Part model, mm, in its own coordinate system. Face numbers are marked on the shaded views. A direction names the side the tool comes from. Coordinates: 2 decimals unless noted, no trailing zeros. Write each loop counter-clockwise with the first axis right and the second up, starting at its lowest first coordinate (ties: lowest second). Pieces come first, ordered by that corner, then holes. Notation, with made-up numbers: M 19,0.5 L 51,0.5 A14 ccw 51,17.5 Z; hole C 79,8 d10. An arc over 180 degrees is marked long. Use a Markdown table: item, result. Add a question column.
Q1. Pin check, flat tip, straight feed: pin 1 Ø4 at (x, y) = (4.57, 10.04) entering from +Z. Stop position of the tip, or through.
Q2. Slice it at A-A on y = 2.96. Write the cut outline in (x, z).
Q3. Slice it at C-C on y = 22.61. Write the cut outline in (x, z).
Q4. Slice it at B-B on z = -1.7. Write the cut outline in (x, y).
Q5. Slice it at D-D on z = -0.35. Write the cut outline in (x, y), then the cut area to 3 significant figures.
Q6. Mould opens along Y. For the marked faces 3, 4, 5 and 6 say: released by +Y, released by -Y, zero draft, split by the parting line, or undercut.
Q7. Tool access for the marked faces 1 and 2: list every direction of +Z, -Z, +X, -X, +Y, -Y with a clear straight run to the whole face (end or side of a thin tool).
Q8. Wall check: L1, parallel to X at y = 11.75, z = -0.3; L2, parallel to X at y = 22.5, z = -1.75; L3, parallel to Y at x = 15, z = -1.65. Give the ranges that are in metal, low to high. Write a range as from..to.
from build123d import *

# Parameters (mm, degrees)
SKETCH1_W                                       = 20
SKETCH1_H                                       = 29.11
SKETCH1_R                                       = 1.5
SKETCH1_R_2                                     = 1.2
SKETCH1_R_3                                     = 5
BOSS_EXTRUDE2_DEPTH                             = 3.18
CSK_FOR_M2_FLAT_HEAD_MACHINE_SCREW1_D           = 2.4
CSK_FOR_M2_FLAT_HEAD_MACHINE_SCREW1_DEPTH       = 3.508967257
CSK_FOR_M2_FLAT_HEAD_MACHINE_SCREW1_CSINK_D     = 4.4
CSK_FOR_M2_FLAT_HEAD_MACHINE_SCREW1_CSINK_ANGLE = 90
CSK_FOR_M2_FLAT_HEAD_MACHINE_SCREW1_TIP         = 0.721032743
CHAMFER1_SIZE                                   = 1.8
FILLET1_R                                       = 0.5
CUT_EXTRUDE1_DEPTH                              = 4
FILLET6_R                                       = 0.5
CUT_EXTRUDE2_DEPTH                              = 4
FILLET8_R                                       = 1


with BuildPart() as part:
    # Sketch1 → Boss-Extrude2 (new body)
    with BuildSketch(Plane.XY):
        with Locations((10, 14.555)):
            Rectangle(SKETCH1_W, SKETCH1_H)
        with Locations((5, 22.61)):
            Circle(SKETCH1_R, mode=Mode.SUBTRACT)
        with Locations((15, 24.61)):
            Circle(SKETCH1_R, mode=Mode.SUBTRACT)
        with Locations((15.03, 14.21)):
            Circle(SKETCH1_R_2, mode=Mode.SUBTRACT)
        with Locations((4.57, 10.04)):
            Circle(SKETCH1_R_2, mode=Mode.SUBTRACT)
        with Locations((13.41, 2.96)):
            Circle(SKETCH1_R_2, mode=Mode.SUBTRACT)
        with Locations((11, 9.11)):
            Circle(SKETCH1_R_3, mode=Mode.SUBTRACT)
    extrude(amount=-BOSS_EXTRUDE2_DEPTH)

    # CSK for M2 Flat Head Machine Screw1
    with Locations(Plane.XY):
        with Locations((4.57, 10.04), (15.03, 14.21), (13.41, 2.96)):
            CounterSinkHole(CSK_FOR_M2_FLAT_HEAD_MACHINE_SCREW1_D / 2, CSK_FOR_M2_FLAT_HEAD_MACHINE_SCREW1_CSINK_D / 2, depth=CSK_FOR_M2_FLAT_HEAD_MACHINE_SCREW1_DEPTH, counter_sink_angle=CSK_FOR_M2_FLAT_HEAD_MACHINE_SCREW1_CSINK_ANGLE)
            with Locations((0, 0, -(CSK_FOR_M2_FLAT_HEAD_MACHINE_SCREW1_DEPTH + CSK_FOR_M2_FLAT_HEAD_MACHINE_SCREW1_TIP / 2))):  # 118° drill point
                Cone(0, CSK_FOR_M2_FLAT_HEAD_MACHINE_SCREW1_D / 2, CSK_FOR_M2_FLAT_HEAD_MACHINE_SCREW1_TIP, mode=Mode.SUBTRACT)

    # Chamfer1
    chamfer1_edges = [part.edges().sort_by_distance(p)[0] for p in [
        (0, 29.11, -1.59),
        (20, 29.11, -1.59),
    ]]
    chamfer(chamfer1_edges, length=CHAMFER1_SIZE)

    # Fillet1
    fillet1_edges = [part.edges().sort_by_distance(p)[0] for p in [
        (0, 27.31, -1.59),
        (20, 27.31, -1.59),
    ]]
    fillet(fillet1_edges, radius=FILLET1_R)

    # Sketch12 → Cut-Extrude1 (cut)
    with BuildSketch(Plane(origin=(0, 0, -3.18), x_dir=(-1, 0, 0), z_dir=(0, 0, -1))):
        Polygon((0, 0), (-20, 0), (-20, 1.60680291), (-15.748577863, 1.60680291), (-13.898929975, 0.251358625), (0, 0.251358625), align=None)
    extrude(amount=-CUT_EXTRUDE1_DEPTH, mode=Mode.SUBTRACT)

    # Fillet6
    fillet6_edges = [part.edges().sort_by_distance(p)[0] for p in [
        (0, 0.251358625, -1.59),
        (20, 1.60680291, -1.59),
        (15.748577863, 1.60680291, -1.59),
    ]]
    fillet(fillet6_edges, radius=FILLET6_R)

    # Sketch14 → Cut-Extrude2 (cut)
    with BuildSketch(Plane.XY):
        Polygon((12.898929975, 0.251358625), (13.898929975, 0.251358625), (14.705535433, 0.842448835), align=None)
    extrude(amount=-CUT_EXTRUDE2_DEPTH, mode=Mode.SUBTRACT)

    # Fillet8
    fillet8_edges = [part.edges().sort_by_distance(p)[0] for p in [
        (12.898929975, 0.251358625, -1.59),
        (14.705535433, 0.842448835, -1.59),
    ]]
    fillet(fillet8_edges, radius=FILLET8_R)


solid = part.part
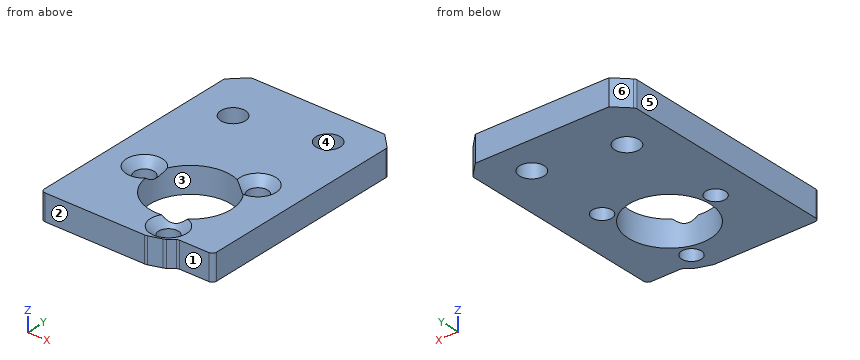
Recorded:
| question | item | result |
|---|---|---|
| 1 | pin 1 | z = -0.2 |
| 2 | outline | M 0,-3.18 L 12.21,-3.18 L 12.21,-1 L 11.21,0 L 0,0 Z; M 14.61,-3.18 L 20,-3.18 L 20,0 L 15.61,0 L 14.61,-1 Z |
| 3 | outline | M 0,-3.18 L 3.5,-3.18 L 3.5,0 L 0,0 Z; M 6.5,-3.18 L 20,-3.18 L 20,0 L 6.5,0 Z |
| 4 | outline | M 0,0.75 A0.5 ccw 0.5,0.25 L 12.74,0.25 A1 ccw 13.05,0.3 L 14.55,0.79 A1 ccw 14.83,0.94 L 15.62,1.51 A0.5 cw 15.91,1.61 L 19.5,1.61 A0.5 ccw 20,2.11 L 20,27.1 A0.5 ccw 19.85,27.46 L 18.2,29.11 L 1.8,29.11 L 0.15,27.46 A0.5 ccw 0,27.1 Z; hole C 4.57,10.04 d2.4; hole C 5,22.61 d3; hole C 11,9.11 d10; hole C 13.41,2.96 d2.4; hole C 15,24.61 d3; hole C 15.03,14.21 d2.4 |
| 5 | outline | M 0,0.75 A0.5 ccw 0.5,0.25 L 12.74,0.25 A1 ccw 13.05,0.3 L 14.55,0.79 A1 ccw 14.83,0.94 L 15.62,1.51 A0.5 cw 15.91,1.61 L 19.5,1.61 A0.5 ccw 20,2.11 L 20,27.1 A0.5 ccw 19.85,27.46 L 18.2,29.11 L 1.8,29.11 L 0.15,27.46 A0.5 ccw 0,27.1 Z; hole C 5,22.61 d3; hole M 6.01,8.87 A5 ccw 12.06,4.22 A1.85 ccw long 13.54,4.81 A5 ccw 14.79,12.38 A1.85 ccw long 13.3,13.55 A5 ccw 6.28,10.75 A1.85 ccw long Z; hole C 15,24.61 d3 |
| 5 | area | 443 mm² |
| 6 | face 3 | undercut |
| 6 | face 4 | undercut |
| 6 | face 5 | zero draft |
| 6 | face 6 | released by +Y |
| 7 | face 1 | +Z, -Z, +X, -Y |
| 7 | face 2 | +Z, -Z, +X, -X, -Y |
| 8 | L1 | 0..3.74, 5.4..6.75, 15.25..20 |
| 8 | L2 | 0..3.5, 6.5..20 |
| 8 | L3 | 1.06..6.11, 12.11..13.01, 15.41..23.11, 26.11..29.11 |
